Autodesk Inventor part; units mm, degrees
ref_plane "YZ Plane" through (0, 0, 0) normal (1, 0, 0) x (0, 1, 0)
ref_plane "XZ Plane" through (0, 0, 0) normal (0, 1, 0) x (-1, 0, 0)
ref_plane "XY Plane" through (0, 0, 0) normal (0, 0, 1) x (1, 0, 0)
sketch "Sketch1" plane through (0, 0, 0) normal (0, 0, 1) x (1, 0, 0)
  line L0 (-2.5, 100) -> (2.5, 100)
  line L1 (2.5, 100) -> (2.5, 0)
  line L2 (2.5, 0) -> (-2.5, 0)
  line L3 (-2.5, 0) -> (-2.5, 100)
  line L4 (0, -20) -> (0, 120)
  line L5 (-3.5, 0) -> (3.5, 0)
  point P0 (0, 0)
  point P1 (0, 100)
  dimension "d0" = 5
  dimension "d1" = 100
extrude "Extrusion1" add sketch "Sketch1" along normal mid plane 14
sketch "Sketch2" plane through (-2.5, 100, 7) normal (0, 1, 0) x (1, 0, 0)
  line L0 (5, 0) -> (0, 0)
  line L1 (0, 0) -> (12, 0)
  line L2 (12, 0) -> (12, 14)
  line L3 (12, 14) -> (0, 14)
  line L4 (0, 14) -> (0, 0)
  line L5 (0, 14) -> (5, 14)
  line L6 (5, 14) -> (5, 0)
  point P0 (2.5, 7)
  dimension "d5" = 7
extrude "Extrusion2" add sketch "Sketch2" against normal blind 3
sketch "Sketch3" plane through (-2.5, 100, 7) normal (0, 1, 0) x (1, 0, 0)
  line L0 (12, 0) -> (12, 14)
  line L1 (0, 14) -> (12, 14)
  line L2 (0, 0) -> (12, 0)
  point P0 (2.5, 7)
  point P1 (9, 2)
  point P2 (9, 12)
  dimension "d8" = 3
  dimension "d9" = 2
  dimension "d10" = 2
hole "Hole1" at (6.5, 100, 5) at (6.5, 100, -5) direction (0, -1, 0) diameter 3.4 end through all
sketch "Sketch4" plane through (-2.5, 0, 7) normal (0, -1, 0) x (1, 0, 0)
  line L0 (-8, 0) -> (13, 0)
  line L1 (13, 0) -> (13, -14)
  line L2 (13, -14) -> (-8, -14)
  line L3 (-8, -14) -> (-8, 0)
  line L4 (0, 0) -> (5, 0)
  line L5 (5, -14) -> (0, -14)
  line L6 (0, -14) -> (0, 0)
  line L7 (12, -14) -> (12, 0)
  line L8 (5, 0) -> (5, -14)
  point P0 (2.5, -7)
  dimension "d18" = 8
  dimension "d20" = 8
extrude "Extrusion3" add sketch "Sketch4" against normal blind 3
sketch "Sketch5" plane through (-2.5, 3, 7) normal (0, 1, 0) x (1, 0, 0)
  line L0 (-4.5, 11) -> (-4.5, 3) construction
  line L1 (-8, 14) -> (-8, 0) construction
  point P0 (2.5, 7)
  point P1 (-4.5, 7)
  point P2 (-8, 7)
  dimension "d23" = 8
  dimension "d24" = 3.5
hole "Hole2" at (-7, 3, -4) at (-7, 3, 4) direction (0, -1, 0) diameter 3.4 end through all
chamfer "Chamfer1" distance 8 angle 45 1 edges at (2.5, 3, 0)
chamfer "Chamfer2" distance 1 angle 45 1 edges at (-2.5, 3, 0)
properties part number "compass mount"
Here's how the part is built. I have some questions about the finished solid (model axes, mm). A direction names the side the tool comes from. Round coordinates to 2 decimals unless told otherwise and drop trailing zeros. Order: outer loops, then holes, each group sorted by start corner. A loop starts at its lowest first (then second) coordinate and runs counter-clockwise, first axis right, second up. Notation, with made-up numbers: M 13,40 L 19,40 A13 ccw 19,65 Z; hole C 73.25,-29.5 d8. An arc over 180 degrees is marked long. Return JSON: item names as keys, results as strings. Group by question number.
1. Please list where these lines run through material, in increasing order: probe 1 along Z at (x, y) = (-7, 1.4); probe 2 along Z at (x, y) = (6.5, 99); probe 3 along X at (y, z) = (2.3, -4).
2. I'm going to push flat-ended pins straight in: pin 1 Ø2.5 at (x, z) = (6.5, 5) entering from +Y; pin 2 Ø2 at (x, z) = (-8, 3.5) entering from +Y; pin 3 Ø8 at (y, z) = (13, 3.5) entering from +X. Where does each tip first touch, or does it pass through?
3. If we section it at B-B on x = -7: List the corners of the cut face in (y, z) for me.
4. If we section it at C-C on x = 6.5: List the corners of the cut face in (y, z) for me, then the cut area to 3 significant figures.
5. If we section it at A-A on z = 4.25: State how many separate pieces and enclosed holes the cut face has, then the cut area to 3 significant figures.
6. If we mould it in two halves opening along Z, with no side actions, what happens to faces 1 (the face through (6.4, 7.1, 0.1)), 2 (the face through (0, 47, -7)), 3 (the face through (-5.5, 1.5, -3.2)), 4 (the face through (-5.5, 1.5, 4.8))? For each: pulls with the +Z half, pulls with the -Z half, needs draft (parallel to the pull), parting line crosses it, or undercut.
7. On a 3-axis mill with a long thin cutter (end or side, diameter ignored), from which of +Z, -Z, +X, -X, +Y, -Y can I reach the whole of each face in a straight line? I mean faces 5 (the face through (-2.5, 51, 0)), 6 (the face through (6, 97, 0)), 7 (the face through (8, 98.5, 5.8)), 8 (the face through (9.5, 99, 0)), 9 (the face through (0, 0, 0)). Say none if no direction works.
Reply:
{
 "1": {"probe 1": "-7 to -5.7, -2.3 to 2.3, 5.7 to 7", "probe 2": "-7 to -6.7, -3.3 to 3.3, 6.7 to 7", "probe 3": "-10.5 to -8.7, -5.3 to 10.5"},
 "2": {"pin 1": "y = 8.25", "pin 2": "y = 3", "pin 3": "x = 4.5"},
 "3": {"outline": "M 0,-7 L 3,-7 L 3,-5.7 L 0,-5.7 Z; M 0,-2.3 L 3,-2.3 L 3,2.3 L 0,2.3 Z; M 0,5.7 L 3,5.7 L 3,7 L 0,7 Z"},
 "4": {"outline": "M 0,-7 L 7,-7 L 7,7 L 0,7 Z; M 97,-7 L 100,-7 L 100,-6.7 L 97,-6.7 Z; M 97,-3.3 L 100,-3.3 L 100,3.3 L 97,3.3 Z; M 97,6.7 L 100,6.7 L 100,7 L 97,7 Z", "area": "120 mm^2"},
 "5": {"separate pieces": "3", "enclosed holes": "0", "area": "582 mm^2"},
 "6": {"face 1": "needs draft", "face 2": "pulls with the -Z half", "face 3": "undercut", "face 4": "undercut"},
 "7": {"face 5": "+Z, -Z, -X, +Y", "face 6": "+Z, -Z, +X", "face 7": "+Y", "face 8": "+Z, -Z, +X, +Y", "face 9": "+Z, -Z, +X, -X, -Y"}
}
